Geometry: final body of the model. Coordinates: model frame, mm. A direction names the side the tool comes from. Give positions to 0.01 mm unless a question says otherwise; leave off trailing zeros. Write each loop counter-clockwise with the first axis right and the second up, starting at its lowest first coordinate (ties: lowest second). Pieces come first, ordered by that corner, then holes. Notation, with made-up numbers: M -2,-29.75 L 23,-29.75 A6 ccw 23,-18.75 Z; hole C 9.25,51.5 d6. An arc over 180 degrees is marked long. Use a Markdown table: item, result. Add a question column.
(1) Material intervals for L1, parallel to Y at x = -23.5, z = -64; L2, parallel to Y at x = 9, z = -37, sorted ascending.
(2) Cut plane A-A (z = -57). Output: boundary loops of the cut face in (x, y).
(3) Cut plane B-B (x = 22). Output: boundary loops of the cut face in (y, z).
(4) Pin query (flat end, axial travel): pin 1 Ø3 at (x, z) = (3, -52.5) entering from +Y; pin 2 Ø4 at (x, z) = (-17.5, -59.5) entering from -Y; pin 3 Ø1.2 at (y, z) = (-0.5, -36) entering from -X. Return the tip coordinate at first contact, or that it passes through.
(5) Reachability of faces 1 (the flat face through (1, -0.2, -57)), 2 (the flat face through (11.309, 0, -35)), 3 (the flat face through (1, 0.2, -57)) from +Z, -Z, +X, -X, +Y, -Y: full face, straight path, thin tool, end or side. Return the list, or none.
(6) Draft query along Z for faces 4 (the cylindrical face through (29.705, 0.003, -39.002)), 5 (the flat face through (1, 0.2, -30)), 6 (the cylindrical face through (1.88, 0, -29.54)). Return one class per face: released by +Z, released by -Z, zero draft, split by the parting line, or undercut.
```python
from build123d import *

# Parameters (mm, degrees)
SKETCH_2_R           = 1.25
EXTRUDE_1_DEPTH      = 0.2
EXTRUDE_1_DEPTH_BACK = 0.2
SKETCH_4_R           = 2
EXTRUDE_3_DEPTH      = 0.1
EXTRUDE_3_DEPTH_BACK = 20.1
SKETCH_6_R           = 2.2
SKETCH_6_R_2         = 2
CUT_EXTRUDE_2_DEPTH  = 6
SKETCH_7_R           = 2.2
SKETCH_7_R_2         = 2
CUT_EXTRUDE_3_DEPTH  = 6


with BuildPart() as part:
    # Sketch 2 → Extrude 1 (new body, two sides)
    with BuildSketch(Plane(origin=(0, 0, 0), x_dir=(1, 0, 0), z_dir=(0, 1, 0))) as extrude_1_sk:
        with BuildLine():
            Line((-23.791283512, 37.576059538), (-8.791283512, 37.576059538))
            Line((-8.791283512, 37.576059538), (-8.791283512, 28.485605042))
            ThreePointArc((-8.791283512, 28.485605042), (-7.912603856, 26.364284699), (-5.791283512, 25.485605042))
            Line((-5.791283512, 25.485605042), (8.208716488, 25.485605042))
            ThreePointArc((8.208716488, 25.485605042), (10.330036831, 26.364284699), (11.208716488, 28.485605042))
            Line((11.208716488, 28.485605042), (11.208716488, 37.576059538))
            Line((11.208716488, 37.576059538), (26.208716488, 37.576059538))
            ThreePointArc((26.208716488, 37.576059538), (29.744250394, 39.040525632), (31.208716488, 42.576059538))
            Line((31.208716488, 42.576059538), (31.208716488, 60.485605042))
            ThreePointArc((31.208716488, 60.485605042), (26.815318205, 71.09220676), (16.208716488, 75.485605042))
            Line((16.208716488, 75.485605042), (-13.791283512, 75.485605042))
            ThreePointArc((-13.791283512, 75.485605042), (-24.399223726, 71.093545256), (-28.791283512, 60.485605042))
            Line((-28.791283512, 60.485605042), (-28.791283512, 42.576059538))
            ThreePointArc((-28.791283512, 42.576059538), (-27.326817418, 39.040525632), (-23.791283512, 37.576059538))
        make_face()
        with Locations((1.208716488, 28.485605042)):
            Circle(SKETCH_2_R, mode=Mode.SUBTRACT)
    extrude(amount=EXTRUDE_1_DEPTH)
    extrude(extrude_1_sk.sketch, amount=-EXTRUDE_1_DEPTH_BACK)

    # Sketch 4 → Extrude 3 (add, two sides)
    with BuildSketch(Plane(origin=(11.208716488, 0, 0), x_dir=(0, 0, -1), z_dir=(1, 0, 0))) as extrude_3_sk:
        with Locations((35.376059538, 0)):
            Circle(SKETCH_4_R)
    extrude(amount=EXTRUDE_3_DEPTH)
    extrude(extrude_3_sk.sketch, amount=-EXTRUDE_3_DEPTH_BACK)

    # Sketch 6 → Cut-Extrude 2 (cut)
    with BuildSketch(Plane.ZY.offset(8.891283512)):
        with Locations((-35.376059538, 0)):
            Circle(SKETCH_6_R)
        with Locations((-35.376059538, 0)):
            Circle(SKETCH_6_R_2, mode=Mode.SUBTRACT)
    extrude(amount=-CUT_EXTRUDE_2_DEPTH, mode=Mode.SUBTRACT)

    # Sketch 7 → Cut-Extrude 3 (cut)
    with BuildSketch(Plane(origin=(11.308716488, 0, 0), x_dir=(0, 0, -1), z_dir=(1, 0, 0))):
        with Locations((35.376059538, 0)):
            Circle(SKETCH_7_R)
        with Locations((35.376059538, 0)):
            Circle(SKETCH_7_R_2, mode=Mode.SUBTRACT)
    extrude(amount=-CUT_EXTRUDE_3_DEPTH, mode=Mode.SUBTRACT)


solid = part.part
```
Answer list:
| question | item | result |
|---|---|---|
| 1 | L1 | -0.2 to 0.2 |
| 1 | L2 | -1.17 to 1.17 |
| 2 | outline | M -28.79,-0.2 L 31.21,-0.2 L 31.21,0.2 L -28.79,0.2 Z |
| 3 | outline | M -0.2,-74.32 L 0.2,-74.32 L 0.2,-37.58 L -0.2,-37.58 Z |
| 4 | pin 1 | y = 0.2 |
| 4 | pin 2 | y = -0.2 |
| 4 | pin 3 | x = -8.89 |
| 5 | face 1 | -Z, +X, -X, -Y |
| 5 | face 2 | +Z, +X, +Y, -Y |
| 5 | face 3 | -Z, +X, -X, +Y |
| 6 | face 4 | released by +Z |
| 6 | face 5 | zero draft |
| 6 | face 6 | undercut |
